from build123d import *

# Parameters (mm, degrees)
PAD_DEPTH     = 100
SKETCH002_W   = 16.341032
SKETCH002_H   = 27.015066
SKETCH002_W_2 = 6.216697
SKETCH002_H_2 = 7.460034
POCKET_DEPTH  = 5


with BuildPart() as part:
    # Sketch → Pad (new body)
    with BuildSketch(Plane.XZ):
        Polygon((-30.131472, 0), (-30.131472, 39.766136), (0, 69.846497), (30.080984, 40.183968), (30.080984, 0), align=None)
    extrude(amount=PAD_DEPTH)

    # Sketch002 (on Face7 of Pad) → Pocket (cut)
    with BuildSketch(Plane.XZ.offset(100)):
        with Locations((-11.944406, 13.507533)):
            Rectangle(SKETCH002_W, SKETCH002_H)
        Polygon((-27.042097, 39.981319), (27.664824, 39.981319), (-0.576733, 67.512398), align=None)
        Polygon((7.060923, 28.968885), (7.060923, 20.443129), (12.922381, 20.443129), (13.277617, 28.968885), align=None)
        Polygon((16.474777, 28.968885), (16.474777, 19.555031), (21.625753, 19.555031), (21.625753, 29.324125), align=None)
        Polygon((7.060923, 16.357872), (7.416164, 9.253077), (13.9881, 9.253077), (13.9881, 16.713112), align=None)
        with Locations((19.050264, 13.160713)):
            Rectangle(SKETCH002_W_2, SKETCH002_H_2)
    extrude(amount=-POCKET_DEPTH, mode=Mode.SUBTRACT)


solid = part.part
Read the model definition and answer for the solid it produces. Units are mm, in the model's axes. A direction names the side the tool comes from. Round coordinates to 2 decimals unless told otherwise and drop trailing zeros. Write each loop counter-clockwise with the first axis right and the second up, starting at its lowest first coordinate (ties: lowest second). Pieces come first, ordered by that corner, then holes.
1. The part is cut by section C-C, the plane y = -12.5. Determine the outline of the cut face in (x, z).
2. The part is cut by section D-D, the plane x = -9.5. Determine the outline of the cut face in (y, z), then the cut area to 3 significant figures.
3. Straight lines are drawn through the part: L1, parallel to Y at x = 10.5, z = 15; L2, parallel to Z at x = 8, y = -51.5; L3, parallel to X at y = -89, z = 67.5. For each, find the intervals that lie inside material, in ascending order.
4. Which of the six approach directions +Z, -Z, +X, -X, +Y, -Y give full straight-line access (tool end or side, diameter ignored) to faces 4 (the face through (-12, -95, 14)), 5 (the face through (10.573, -97.535, 16.538))?
5. Determine the mould class of faces 1 (the face through (14.83, -49.3, 55.22)), 2 (the face through (-12, -98, 27.015)), 3 (the face through (19, -98, 9.431)) for opening direction Z: pulls with the +Z half, pulls with the -Z half, needs draft (parallel to the pull), parting line crosses it, or undercut.
6. Given pin 1 Ø10 at (x, y) = (-14.5, -53.5) entering from +Z; pin 2 Ø8 at (x, z) = (-10, 15) entering from -Y; pin 3 Ø1 at (x, y) = (-18, -75) entering from +Z, each flat-ended and moving along its own axis, determine where each tip first touches the part or whether it passes through.
7. The part is cut by section A-A, the plane x = 5. Determine the outline of the cut face in (y, z).
8. The part is cut by section B-B, the plane z = 41.5. Determine the outline of the cut face in (x, y), then the cut area to 3 significant figures.
Values:
1. outline: (-30.13, 0) - (30.08, 0) - (30.08, 40.18) - (0, 69.85) - (-30.13, 39.77) - close
2. outline: (-100, 27.02) - (-95, 27.02) - (-95, 0) - (0, 0) - (0, 60.36) - (-100, 60.36) - (-100, 58.23) - (-95, 58.23) - (-95, 39.98) - (-100, 39.98) - close
2. area: 5,810 mm2
3. L1: y = -95 to 0
3. L2: z = 0 to 61.96
3. L3: x = -2.35 to 2.38
4. face 4: -Z, -Y
4. face 5: -Y
5. face 1: pulls with the +Z half
5. face 2: pulls with the -Z half
5. face 3: undercut
6. pin 1: stops at z = 60.36
6. pin 2: stops at y = -95
6. pin 3: stops at z = 52.38
7. outline: (-100, 0) - (0, 0) - (0, 64.92) - (-100, 64.92) - (-100, 62.08) - (-95, 62.08) - (-95, 39.98) - (-100, 39.98) - close
8. outline: (-28.39, -100) - (-25.58, -100) - (-25.58, -95) - (26.11, -95) - (26.11, -100) - (28.75, -100) - (28.75, 0) - (-28.39, 0) - close
8. area: 5,460 mm2
